The listing builds one solid part. Answer for the finished solid, in the listing's coordinates (mm). Face numbers are marked on the shaded views. Give positions to 0.01 mm unless a question says otherwise; leave off trailing zeros. Order: outer loops, then holes, each group sorted by start corner. A loop starts at its lowest first (then second) coordinate and runs counter-clockwise, first axis right, second up. Notation, with made-up numbers: (-38.75, 17) - (-0.75, 17) arc R35 ccw to (-0.75, 52) - close; hole circle Ø7 at (-6.5, 25.25). An arc over 180 degrees is marked (long way). Answer as a JSON object with one key per item and string values. Group by question number.
Q1. A cutting plane is placed at A-A, the plane z = 0. Give the vertices of the cut face in (x, y) (1 decimal).
Q2. Consider line 1 (X direction, y = 5.25, z = 0) (1 decimal); line 2 (X direction, y = 11, z = 0); line 3 (Y direction, x = 19, z = -7.5). Determine where each line is inside the solid, lowest interval first.
Q3. A cutting plane is placed at C-C, the plane y = 10.25. Give the vertices of the cut face in (x, z) (1 decimal).
Q4. A cutting plane is placed at B-B, the plane y = 3. Give the vertices of the cut face in (x, z) (1 decimal).
Q5. Given pin 1 (1 mm diameter, centred on x = -9.5, y = 7, fed in from -Z); pin 2 (12 mm diameter, centred on x = 18.5, z = 5, fed in from +Y); pin 3 (2.5 mm diameter, centred on x = 1, z = -0.5, fed in from +Y), each flat-ended and moving along its own axis, determine where each tip first touches the part or whether it passes through.
Q6. The mould has two halves that part along X. Classify the marked faces 1, 2 and 3: released by +X, released by -X, zero draft, split by the parting line, or undercut.
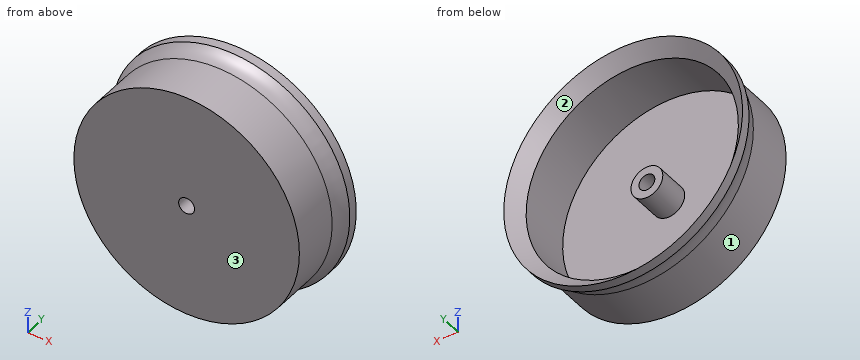
from build123d import *


with BuildPart() as part:
    # Sketch2 → Revolve1 (revolve)
    with BuildSketch(Plane(origin=(0, 0, 0), x_dir=(0, 0, -1), z_dir=(1, 0, 0)), mode=Mode.PRIVATE) as revolve1_sk:
        with BuildLine():
            Line((1.905, 0), (1.905, 9.2075))
            Line((1.905, 9.2075), (3.81, 9.2075))
            Line((3.81, 9.2075), (3.81, 1.5875))
            Line((3.81, 1.5875), (25.4, 1.5875))
            Line((25.4, 1.5875), (25.4, 14.2875))
            Line((25.4, 14.2875), (28.575, 17.4625))
            Line((28.575, 17.4625), (28.575, 15.21743597))
            ThreePointArc((28.575, 15.21743597), (27.400077808, 13.459040646), (26.9875, 11.384871939))
            Line((26.9875, 11.384871939), (26.9875, 0))
            Line((26.9875, 0), (1.905, 0))
        make_face()
    revolve(revolve1_sk.sketch.rotate(Axis((0, 0, 0), (0, -1, 0)), 180), axis=Axis((0, 0, 0), (0, -1, 0)))


solid = part.part
Reply:
{
 "1": {"outline": "(-28.6, 15.2) arc R5.4 cw to (-27, 11.4) - (-27, 0) - (-1.9, 0) - (-1.9, 9.2) - (-3.8, 9.2) - (-3.8, 1.6) - (-25.4, 1.6) - (-25.4, 14.3) - (-28.6, 17.5) - close; (1.9, 0) - (27, 0) - (27, 11.4) arc R5.4 cw to (28.6, 15.2) - (28.6, 17.5) - (25.4, 14.3) - (25.4, 1.6) - (3.8, 1.6) - (3.8, 9.2) - (1.9, 9.2) - close"},
 "2": {"line 1": "x = -27 to -25.4, -3.8 to -1.9, 1.9 to 3.8, 25.4 to 27", "line 2": "x = -26.99 to -25.4, 25.4 to 26.99", "line 3": "y = 0 to 1.59"},
 "3": {"outline": "circle Ø54 at (0, 0); hole circle Ø50.8 at (0, 0)"},
 "4": {"outline": "circle Ø54 at (0, 0); circle Ø7.6 at (0, 0); hole circle Ø50.8 at (0, 0); hole circle Ø3.8 at (0, 0)"},
 "5": {"pin 1": "stops at z = -25.44", "pin 2": "stops at y = 1.59", "pin 3": "stops at y = 9.21"},
 "6": {"face 1": "split by the parting line", "face 2": "undercut", "face 3": "zero draft"}
}
